```python
from build123d import *

# Parameters (mm, degrees)
FILLET_1_R = 0.8
FILLET_2_R = 1.5


with BuildPart() as part:
    # Эскиз1 → Повернуть1 (revolve)
    with BuildSketch(Plane.XY, mode=Mode.PRIVATE) as revolve_1_sk:
        Polygon((0, 0), (0, 4), (3.5, 4), (3.5, 2.5), (63.5, 2.5), (63.5, 4), (67, 4), (67, 0), align=None)
    revolve(revolve_1_sk.sketch.rotate(Axis((0, 0, 0), (-1, 0, 0)), 90), axis=Axis((0, 0, 0), (-1, 0, 0)))

    # Скругление1
    fillet_1_edges = [part.edges().sort_by_distance(p)[0] for p in [
        (63.5, 0, 4),
        (3.5, 0, 4),
    ]]
    fillet(fillet_1_edges, radius=FILLET_1_R)

    # Скругление2
    fillet_2_edges = [part.edges().sort_by_distance(p)[0] for p in [
        (67, 0, 4),
        (0, 0, 4),
    ]]
    fillet(fillet_2_edges, radius=FILLET_2_R)


solid = part.part
```
Work out the finished part from the listing and answer in its coordinate system (mm). A direction names the side the tool comes from. Round coordinates to 2 decimals unless told otherwise and drop trailing zeros. Loops run counter-clockwise (first coordinate to the right, second up) from the corner with the lowest first, then second, coordinate; pieces in that order, holes last. Notation, with made-up numbers: (-40, 18) -> (-33, 18) arc R27 cw to (-33, 49) -> close; hole circle Ø7 at (48.5, -21). An arc over 180 degrees is marked (long way). Write each question's results on one line, items separated by ' | '. Start each with the question number.
1. Find the intervals of material crossed by probe 1 along X at (y, z) = (3, -1.5); probe 2 along Y at (x, z) = (12.5, -0.25); probe 3 along X at (y, z) = (-2.25, 1.5), in increasing order. Write a range as from..to.
2. Section A-A (z = 0) is taken. Determine the outline of the cut face in (x, y), plus the area to 3 significant figures.
3. A tool of negligible diameter and unlimited length cuts with its end or side. For faces 4 (the face through (67, 0, 0)), 5 (the face through (33.9, -0.1, 2.5)), from which of +Z, -Z, +X, -X, +Y, -Y can it reach the whole face along a straight path? Write none if from no direction.
4. Given pin 1 Ø4 at (x, z) = (18.5, 2.5) entering from +Y; pin 2 Ø4 at (x, z) = (40.5, -0.5) entering from -Y, each flat-ended and moving along its own axis, determine where each tip first touches the part or whether it passes through.
5. Section C-C (x = 25) is taken. Determine the outline of the cut face in (y, z), plus the area to 3 significant figures.
6. For a pull along X with two mould halves and no side action, classify faces 1 (the face through (2.108, 3.905, 0.867)), 2 (the face through (0, 0, 0)), 3 (the face through (3.5, 2, 2)) as +X half, -X half, draft (parallel to the pull), parting line (faces both ways), or undercut.
Evaluation:
1) probe 1: x = 0.27..3.49, 63.51..66.73 | probe 2: y = -2.49..2.49 | probe 3: x = 0.01..3.5, 63.5..66.99
2) outline: (0, -2.5) arc R1.5 ccw to (1.5, -4) -> (2.7, -4) arc R0.8 ccw to (3.5, -3.2) -> (3.5, -2.5) -> (63.5, -2.5) -> (63.5, -3.2) arc R0.8 ccw to (64.3, -4) -> (65.5, -4) arc R1.5 ccw to (67, -2.5) -> (67, 2.5) arc R1.5 ccw to (65.5, 4) -> (64.3, 4) arc R0.8 ccw to (63.5, 3.2) -> (63.5, 2.5) -> (3.5, 2.5) -> (3.5, 3.2) arc R0.8 ccw to (2.7, 4) -> (1.5, 4) arc R1.5 ccw to (0, 2.5) -> close | area: 354 mm2
3) face 4: +Z, -Z, +X, +Y, -Y | face 5: none
4) pin 1: stops at y = 2.45 | pin 2: stops at y = -2.5
5) outline: circle Ø5 at (0, 0) | area: 19.6 mm2
6) face 1: draft | face 2: -X half | face 3: undercut
